Check sheet for the drawn part. Datum: minimum x, y, z corner. Units: mm. A direction names the side the tool comes from. Coordinates: 2 decimals unless noted, no trailing zeros. Order: outer loops, then holes, each group sorted by start corner. A loop starts at its lowest first (then second) coordinate and runs counter-clockwise, first axis right, second up.
Q1. Thickness scan on line 1 (Z direction, x = 7.5, y = 28.5) (1 decimal); line 2 (X direction, y = 16.5, z = 11); line 3 (Z direction, x = 84.5, y = 9) (1 decimal). Record the ranges inside material, lowest first.
Q2. Cross-section at D-D, the plane y = 3. Record the boundary of the cut face in (x, z) (1 decimal), and give its area (3 significant figures).
Q3. Cross-section at C-C, the plane x = 35.5. Record the boundary of the cut face in (y, z) (1 decimal), and give its area (4 significant figures).
Q4. Set-up check for the marked faces 1, 2 and 3: record each of +Z, -Z, +X, -X, +Y, -Y from which the full face is reachable in a straight line by a thin tool's end or side.
Q5. Cross-section at B-B, the plane y = 13.5. Record the boundary of the cut face in (x, z) (1 decimal), and give its area (3 significant figures).
Q6. Depth check by flat-ended pin: P1, Ø7.5, axis at y = 15, z = 9, coming from the -X side; P2, Ø9, axis at x = 7.62, z = 59.182, coming from the -Y side; P3, Ø3, axis at x = 33.5, y = 31.5, coming from the -Z side; P4, Ø7.5, axis at x = 60.5, z = 8, coming from the +Y side. Enter the tip coordinate at first touch or a pass-through.
Q7. Cross-section at A-A, the plane x = 7.62. Record the boundary of the cut face in (y, z) (1 decimal).
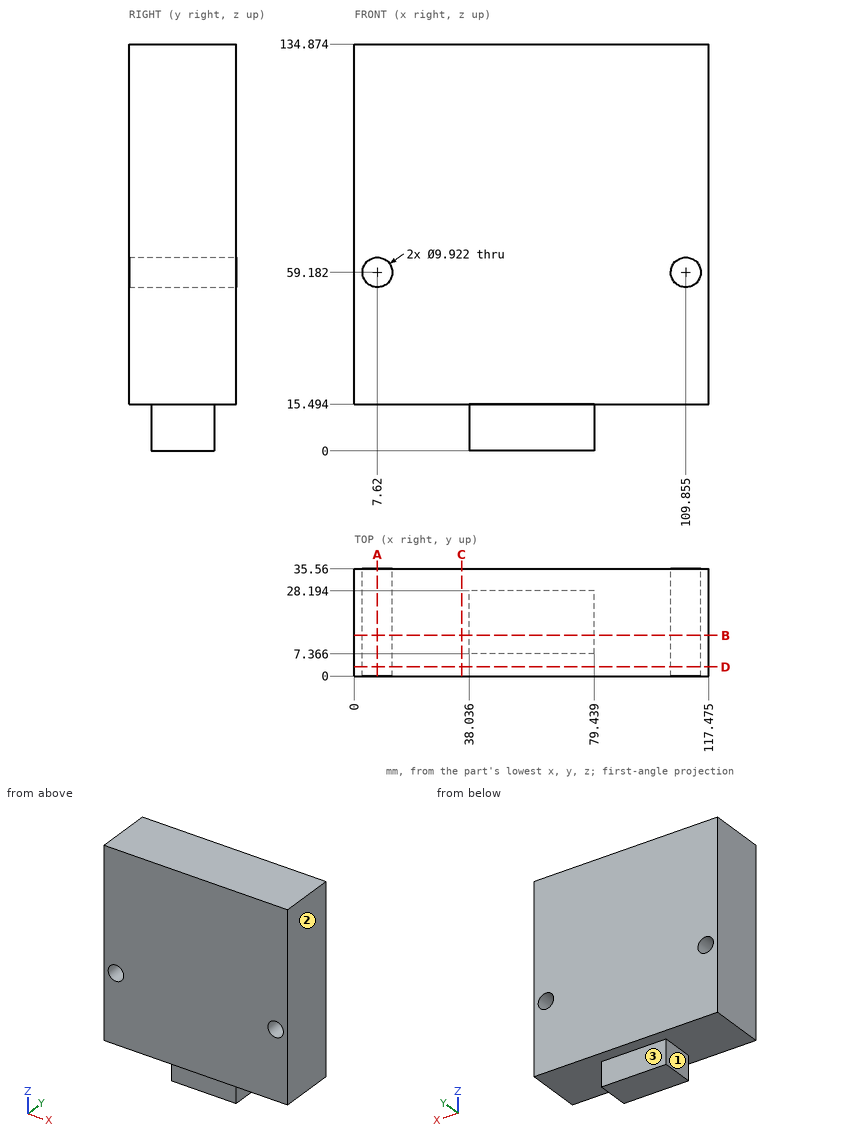
Check values:
1. line 1: z = 15.5 to 54.2, 64.1 to 134.9
1. line 2: x = 38.04 to 79.44
1. line 3: z = 15.5 to 134.9
2. outline: (0, 15.5) - (117.5, 15.5) - (117.5, 134.9) - (0, 134.9) - close; hole circle Ø9.9 at (7.6, 59.2); hole circle Ø9.9 at (109.9, 59.2)
2. area: 13,900 mm2
3. outline: (0, 15.5) - (35.6, 15.5) - (35.6, 134.9) - (0, 134.9) - close
3. area: 4,245 mm2
4. face 1: -Z, -X, +Y, -Y
4. face 2: +Z, -Z, +X, +Y, -Y
4. face 3: -Z, +X, -X, +Y
5. outline: (0, 15.5) - (38, 15.5) - (38, 0) - (79.4, 0) - (79.4, 15.5) - (117.5, 15.5) - (117.5, 134.9) - (0, 134.9) - close; hole circle Ø9.9 at (7.6, 59.2); hole circle Ø9.9 at (109.9, 59.2)
5. area: 14,500 mm2
6. P1: stops at x = 38.04
6. P2: passes through
6. P3: stops at z = 15.49
6. P4: stops at y = 28.19
7. outline: (0, 15.5) - (35.6, 15.5) - (35.6, 54.2) - (0, 54.2) - close; (0, 64.1) - (35.6, 64.1) - (35.6, 134.9) - (0, 134.9) - close
